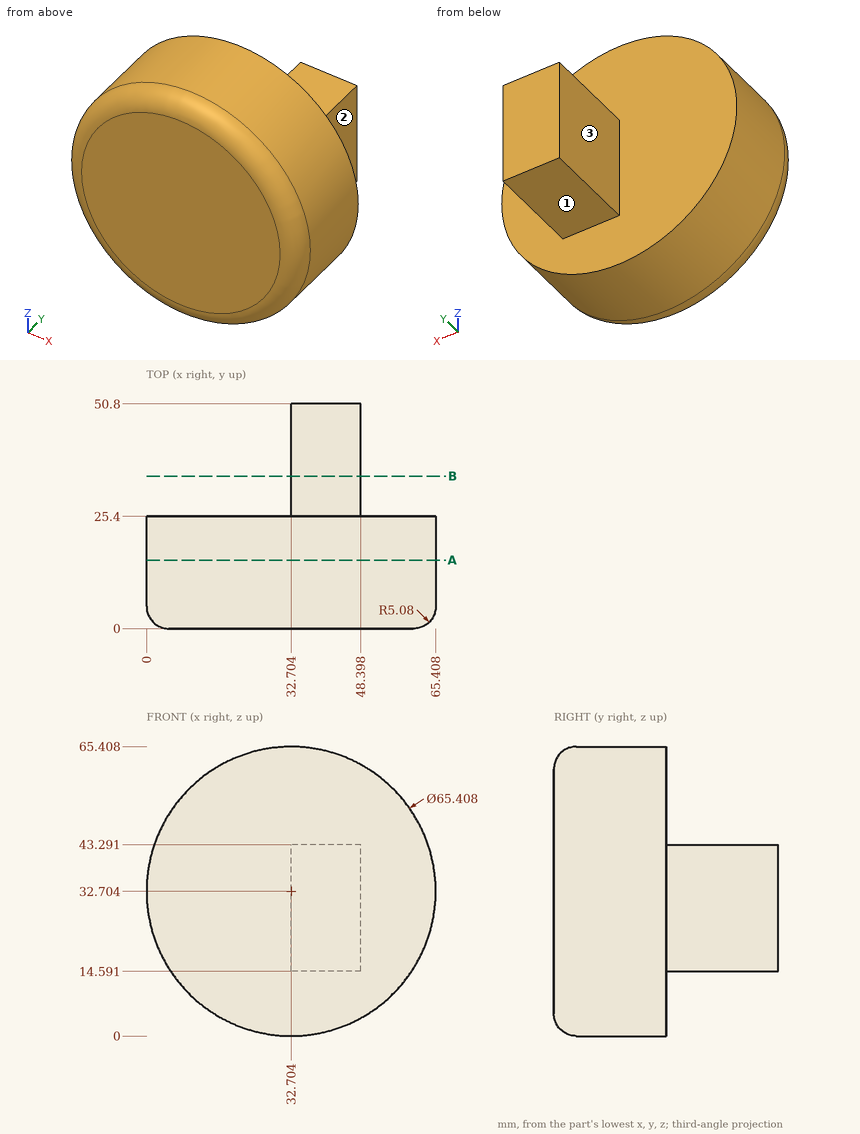
Design review of the part shown in the three views and the two pictorial views. Dimensions are in mm from the part's minimum x, y and z. A direction names the side the tool comes from. Coordinates: 2 decimals unless noted, no trailing zeros. Write each loop counter-clockwise with the first axis right and the second up, starting at its lowest first coordinate (ties: lowest second). Pieces come first, ordered by that corner, then holes.
(1) Tool access review of the marked faces 1, 2 and 3: name each direction out of +Z, -Z, +X, -X, +Y, -Y from which nothing blocks a thin tool from reaching the whole face with its end or side.
(2) Add section A-A on y = 15.5. Give the boundary of the cut face in (x, z), then the cut area to 3 significant figures.
(3) For pin 1 Ø7.5 at (y, z) = (41, 27) entering from -X; pin 2 Ø4 at (x, z) = (32, 12) entering from +Y; pin 3 Ø8 at (x, y) = (28.5, 26) entering from +Z, all flat-tipped, find the tip position at first contact; note any pin that passes through.
(4) Add section B-B on y = 34.5. Give the boundary of the cut face in (x, z).
(5) Wall thickness on probe 1 along Y at (x, z) = (9, 18); probe 2 along Z at (x, y) = (47, 31.5); probe 3 along X at (y, z) = (30, 16.5): over which ranges is each line inside the solid? List them lowest first.
Answer sheet:
1. face 1: -Z, +X, -X, +Y
1. face 2: +Z, -Z, +X, +Y
1. face 3: +Z, -Z, -X, +Y
2. outline: circle Ø65.41 at (32.7, 32.7)
2. area: 3,360 mm2
3. pin 1: stops at x = 32.7
3. pin 2: stops at y = 25.4
3. pin 3: stops at z = 65.41
4. outline: (32.7, 14.59) - (48.4, 14.59) - (48.4, 43.29) - (32.7, 43.29) - close
5. probe 1: y = 0.01 to 25.4
5. probe 2: z = 14.59 to 43.29
5. probe 3: x = 32.7 to 48.4
